Part model, mm, in its own coordinate system. Round coordinates to 2 decimals unless told otherwise and drop trailing zeros. Order: outer loops, then holes, each group sorted by start corner. A loop starts at its lowest first (then second) coordinate and runs counter-clockwise, first axis right, second up. Notation, with made-up numbers: (61, 76) -> (66, 76) arc R34 ccw to (66, 110) -> close; hole circle Ø10 at (55.5, 31). An arc over 180 degrees is marked (long way). Return JSON: item names as keys, results as strings. Group by question number.
from build123d import *

# Parameters (mm, degrees)
SKETCH_W     = 70
SKETCH_H     = 30
PAD_DEPTH    = 2
SKETCH001_R  = 1.5
SKETCH001_W  = 54.5
SKETCH001_H  = 12.5
POCKET_DEPTH = 5


with BuildPart() as part:
    # Sketch → Pad (new body)
    with BuildSketch(Plane.XY):
        Rectangle(SKETCH_W, SKETCH_H)
    extrude(amount=PAD_DEPTH)

    # Sketch001 → Pocket (cut)
    with BuildSketch(Plane.XY):
        with Locations((-30.555, 0)):
            Circle(SKETCH001_R)
        with Locations((30.555, 0)):
            Circle(SKETCH001_R)
        Rectangle(SKETCH001_W, SKETCH001_H)
    extrude(amount=POCKET_DEPTH, mode=Mode.SUBTRACT)


solid = part.part
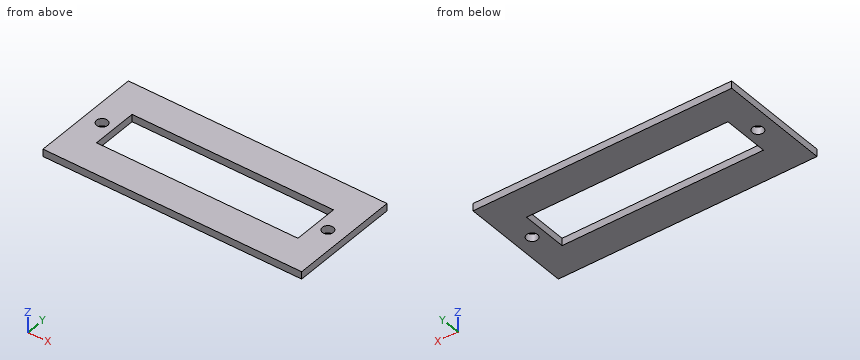
(1) Pin check, flat tips, straight feed: P1, Ø2.5, axis at x = 30.555, y = 0, coming from the -Z side; P2, Ø5, axis at x = -30.555, y = 0, coming from the -Z side. Stop position of each tip, or through.
(2) Saw through at C-C, the plane z = 0.7. List the corners of the cut face in (x, y) (3 decimals), and give its area (3 significant figures).
(3) Probe L1, parallel to X at y = 0, z = 0.95 (3 decimals); L2, parallel to Y at x = -20.5, z = 1.3; L3, parallel to X at y = 2.5, z = 1.8. List the from-to ranges inside material, lowest first. Write a range as [from, to].
(4) Saw through at A-A, the plane y = -5.25. List the corners of the cut face in (x, z), and give its area (3 significant figures).
(5) Saw through at B-B, the plane y = 0. List the corners of the cut face in (x, z) (3 decimals).
Results are:
{
 "1": {"P1": "passes through", "P2": "stops at z = 0"},
 "2": {"outline": "(-35, -15) -> (35, -15) -> (35, 15) -> (-35, 15) -> close; hole circle Ø3 at (-30.555, 0); hole (-27.25, -6.25) -> (27.25, -6.25) -> (27.25, 6.25) -> (-27.25, 6.25) -> close; hole circle Ø3 at (30.555, 0)", "area": "1,400 mm^2"},
 "3": {"L1": "x = [-35, -32.055], [-29.055, -27.25], [27.25, 29.055], [32.055, 35]", "L2": "y = [-15, -6.25], [6.25, 15]", "L3": "x = [-35, -27.25], [27.25, 35]"},
 "4": {"outline": "(-35, 0) -> (-27.25, 0) -> (-27.25, 2) -> (-35, 2) -> close; (27.25, 0) -> (35, 0) -> (35, 2) -> (27.25, 2) -> close", "area": "31.0 mm^2"},
 "5": {"outline": "(-35, 0) -> (-32.055, 0) -> (-32.055, 2) -> (-35, 2) -> close; (-29.055, 0) -> (-27.25, 0) -> (-27.25, 2) -> (-29.055, 2) -> close; (27.25, 0) -> (29.055, 0) -> (29.055, 2) -> (27.25, 2) -> close; (32.055, 0) -> (35, 0) -> (35, 2) -> (32.055, 2) -> close"}
}
